Geometry check sheet. Reference: drawing and pictorial views, mm from the part's lowest x, y, z. A direction names the side the tool comes from. Round coordinates to 2 decimals unless told otherwise and drop trailing zeros. Write each loop counter-clockwise with the first axis right and the second up, starting at its lowest first coordinate (ties: lowest second). Pieces come first, ordered by that corner, then holes. Notation, with made-up numbers: (84, -22) - (112, -22) arc R31 ccw to (112, 8) - close; hole circle Ø2 at (17.25, -27.75). An arc over 180 degrees is marked (long way). Return JSON: item names as keys, results as strings.
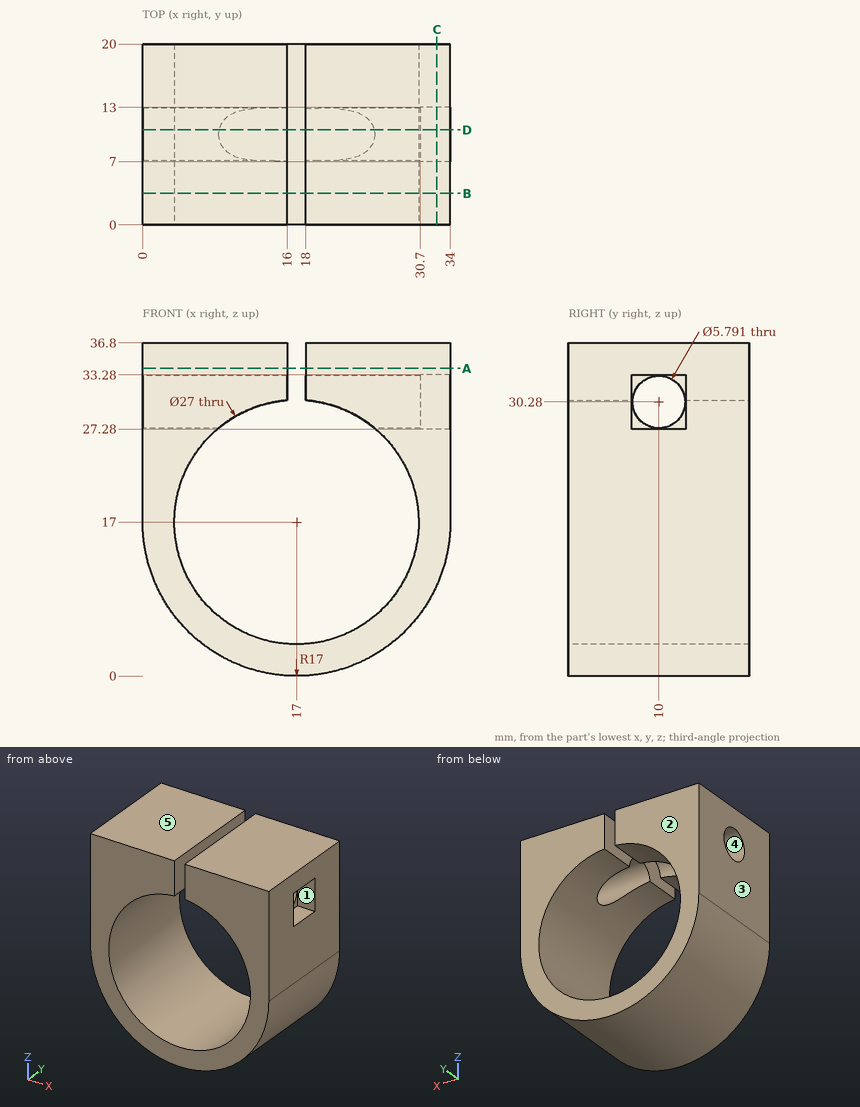
(1) Section check B-B, the plane y = 3.5. Enter the section's corners in (x, z), plus the area to 3 significant figures.
Response values:
{"outline": "(0, 17) arc R17 ccw to (34, 17) - (34, 36.8) - (18, 36.8) - (18, 30.46) arc R13.5 cw (long way) to (16, 30.46) - (16, 36.8) - (0, 36.8) - close", "area": "542 mm^2"}
(2) Release check for a two-part mould opening along Z. For the marked faces 3, 4 and 5 record: pulls with the +Z half, pulls with the -Z half, needs draft (parallel to the pull), parting line crosses it, or undercut.
Response values:
{"face 3": "needs draft", "face 4": "undercut", "face 5": "pulls with the +Z half"}
(3) Section check D-D, the plane y = 10.5. Enter the section's corners in (x, z).
Response values:
{"outline": "(0, 17) arc R17 ccw to (34, 17) - (34, 27.28) - (30.7, 27.28) - (30.7, 27.43) - (25.57, 27.43) arc R13.5 cw (long way) to (8.43, 27.43) - (0, 27.43) - close; (0, 33.13) - (16, 33.13) - (16, 36.8) - (0, 36.8) - close; (18, 33.13) - (30.7, 33.13) - (30.7, 33.28) - (34, 33.28) - (34, 36.8) - (18, 36.8) - close"}
(4) Access from +Z, -Z, +X, -X, +Y, -Y to the whole of each face (thin tool, end or side, straight path). Record for the marked faces 1 and 2.
Response values:
{"face 1": "+X", "face 2": "+Z, -Z, +X, -X, +Y"}
(5) Gauge pin test, flat ends, axial feed: pin 1 (1 mm diameter, centred on x = 33, y = 10, fed in from -Z); pin 2 (1 mm diameter, centred on y = 17, z = 5.5, fed in from +X); pin 3 (5 mm diameter, centred on y = 8.5, z = 30, fed in from +X); pin 4 (8 mm diameter, centred on x = 24.5, y = 13, fed in from -Z). Record the tip position at first contact, or that the pin passes through.
Response values:
{"pin 1": "stops at z = 10.02", "pin 2": "stops at x = 29.96", "pin 3": "stops at x = 34", "pin 4": "stops at z = 0.36"}
(6) Section check C-C, the plane x = 32.5. Enter the section's corners in (y, z).
Response values:
{"outline": "(0, 10.02) - (20, 10.02) - (20, 36.8) - (0, 36.8) - close; hole (7, 27.28) - (13, 27.28) - (13, 33.28) - (7, 33.28) - close"}
(7) Section check A-A, the plane z = 34. Enter the section's corners in (x, y).
Response values:
{"outline": "(0, 0) - (16, 0) - (16, 20) - (0, 20) - close; (18, 0) - (34, 0) - (34, 20) - (18, 20) - close"}
(8) Material ranges on line 1 along X through (y, z) = (11.25, 17); line 2 along Z through (x, y) = (22.75, 10); line 3 along Z through (x, y) = (22.5, 5.75), recorded low to high. Write a range as [from, to].
Response values:
{"line 1": "x = [0, 3.5], [30.5, 34]", "line 2": "z = [1, 4.79], [33.18, 36.8]", "line 3": "z = [0.91, 4.67], [29.33, 36.8]"}
